For this review, take the finished solid that the model builds, in its own axes (mm). Face numbers are marked on the shaded views. A direction names the side the tool comes from. Coordinates: 2 decimals unless noted, no trailing zeros. Order: outer loops, then holes, each group sorted by start corner. A loop starts at its lowest first (then second) coordinate and runs counter-clockwise, first axis right, second up. Notation, with made-up numbers: (86, 3.5) -> (105, 3.5) arc R13 ccw to (105, 11.5) -> close; hole circle Ø7 at (-39, 20.25). An arc over 180 degrees is marked (long way). Answer as a JSON object with one key per item and string values. Group by question number.
1) Add section D-D, the plane z = 17. Write out the cut boundary in (x, y) (3 decimals), then the cut area to 3 significant figures.
2) Add section A-A, the plane x = 0. Write out the cut boundary in (y, z) (3 decimals), then the cut area to 3 significant figures.
3) Add section C-C, the plane y = 18.5. Write out the cut boundary in (x, z).
4) Wall thickness on L1, parallel to Z at x = 0, y = 4 (3 decimals); L2, parallel to X at y = 25.5, z = 0; L3, parallel to X at y = 2, z = 304: over which ranges is each line inside the solid? List them lowest first.
5) Add section B-B, the plane z = 298.5. Write out the cut boundary in (x, y) (3 decimals), then the cut area to 3 significant figures.
6) Machinability: for the marked faces 1 and 2, which of the approach directions +Z, -Z, +X, -X, +Y, -Y give a long, thin tool a straight path to every point of the face, cutting with its end or side? Answer none if there is none.
7) For pin 1 (1 mm diameter, centred on x = -2, y = 19, fed in from -Z); pin 2 (12 mm diameter, centred on x = 18.5, y = 4.5, fed in from -Z), all flat-tipped, find the tip position at first contact; note any pin that passes through.
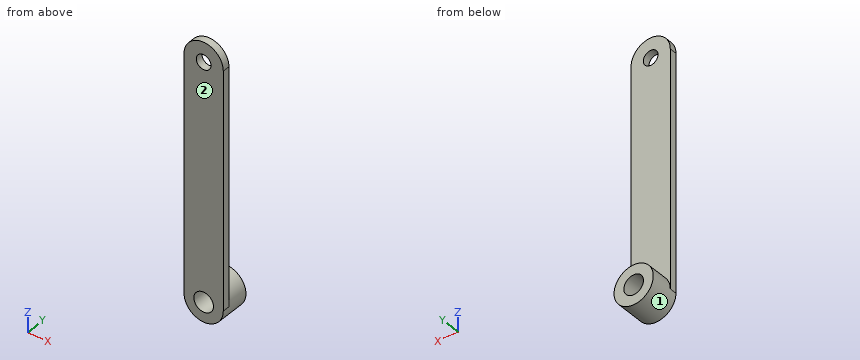
from build123d import *

# Parameters (mm, degrees)
F0_R     = 25.4
F0_R_2   = 12.7
F1_DEPTH = 38.1
F3_DEPTH = 9.525


with BuildPart() as f1:
    # F0 (on Front) → F1 (new body)
    with BuildSketch(Plane.XZ):
        Circle(F0_R)
        Circle(F0_R_2, mode=Mode.SUBTRACT)
    extrude(amount=-F1_DEPTH)

    # F2 (on Front) → F3 (join)
    with BuildSketch(Plane.XZ):
        with BuildLine():
            ThreePointArc((-12.7, 0), (0, 12.7), (12.7, 0))
            Line((12.7, 0), (25.4, 0))
            Line((25.4, 0), (25.4, 304.8))
            Line((25.4, 304.8), (9.525, 304.8))
            ThreePointArc((9.525, 304.8), (0, 295.275), (-9.525, 304.8))
            Line((-9.525, 304.8), (-25.4, 304.8))
            Line((-25.4, 304.8), (-25.4, 0))
            Line((-25.4, 0), (-12.7, 0))
        make_face()
        with BuildLine():
            Line((9.525, 304.8), (25.4, 304.8))
            ThreePointArc((25.4, 304.8), (0, 330.2), (-25.4, 304.8))
            Line((-25.4, 304.8), (-9.525, 304.8))
            ThreePointArc((-9.525, 304.8), (0, 314.325), (9.525, 304.8))
        make_face()
    extrude(amount=-F3_DEPTH)


solid = f1.part
Output values:
{
 "1": {"outline": "(-25.4, 0) -> (25.4, 0) -> (25.4, 9.525) -> (18.872, 9.525) -> (18.872, 38.1) -> (-18.872, 38.1) -> (-18.872, 9.525) -> (-25.4, 9.525) -> close", "area": "1,560 mm²"},
 "2": {"outline": "(0, -25.4) -> (38.1, -25.4) -> (38.1, -12.7) -> (0, -12.7) -> close; (0, 12.7) -> (38.1, 12.7) -> (38.1, 25.4) -> (9.525, 25.4) -> (9.525, 295.275) -> (0, 295.275) -> close; (0, 314.325) -> (9.525, 314.325) -> (9.525, 330.2) -> (0, 330.2) -> close", "area": "3,690 mm²"},
 "3": {"outline": "circle Ø50.8 at (0, 0); hole circle Ø25.4 at (0, 0)"},
 "4": {"L1": "z = -25.4 to -12.7, 12.7 to 295.275, 314.325 to 330.2", "L2": "x = -25.4 to -12.7, 12.7 to 25.4", "L3": "x = -25.4 to -9.49, 9.49 to 25.4"},
 "5": {"outline": "(-25.4, 0) -> (-7.144, 0) -> (-7.144, 9.525) -> (-25.4, 9.525) -> close; (7.144, 0) -> (25.4, 0) -> (25.4, 9.525) -> (7.144, 9.525) -> close", "area": "348 mm²"},
 "6": {"face 1": "+Y", "face 2": "+Z, -Z, +X, -X, -Y"},
 "7": {"pin 1": "stops at z = -25.36", "pin 2": "stops at z = -22.11"}
}
